Check sheet for the drawn part. Datum: minimum x, y, z corner. Units: mm. Round coordinates to 2 decimals unless told otherwise and drop trailing zeros. Order: outer loops, then holes, each group sorted by start corner. A loop starts at its lowest first (then second) coordinate and runs counter-clockwise, first axis right, second up. Notation, with made-up numbers: M 34.25,34 L 60.25,34 A20 cw 60.25,62 Z; hole C 41.25,78 d2. An arc over 180 degrees is marked long. Answer as a JSON object with one key per item and string values. Group by question number.
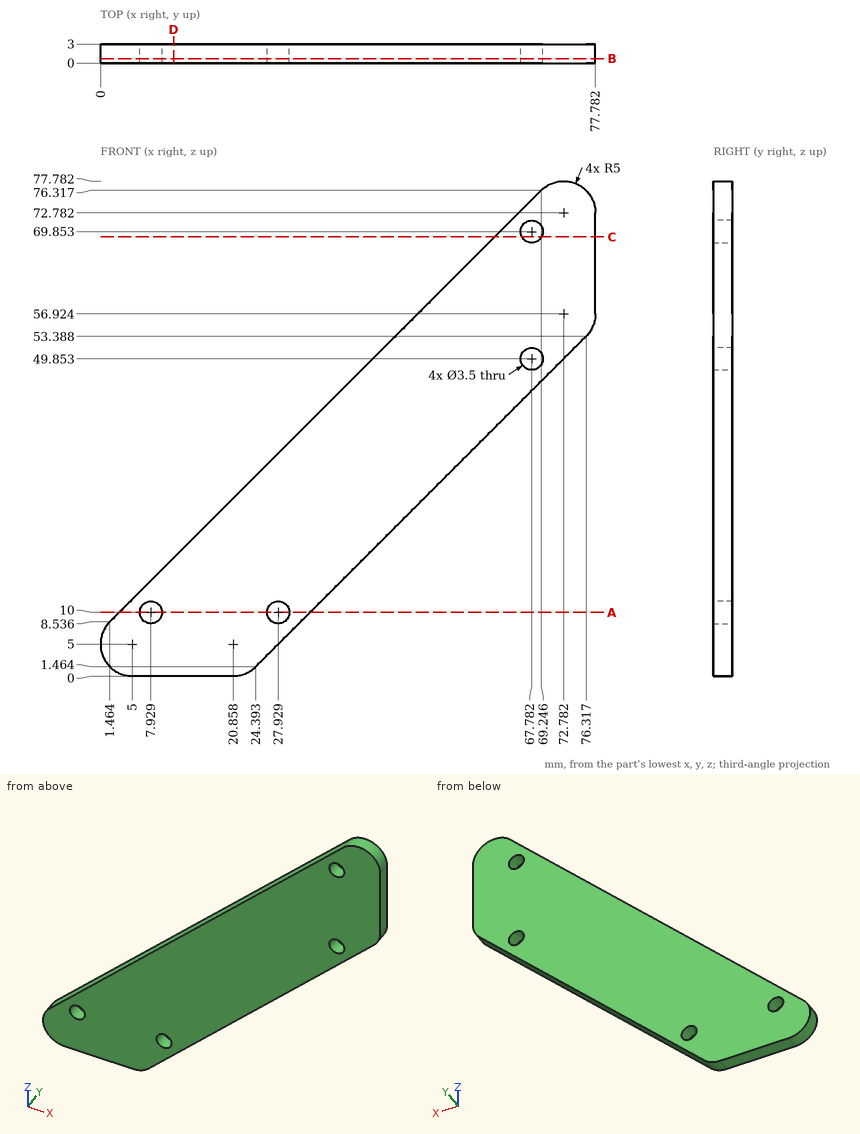
1) Thickness scan on line 1 along X through (y, z) = (1.9, 10); line 2 along Z through (x, y) = (8, 2.05); line 3 along Z through (x, y) = (27, 1.9) (1 decimal). Record the ranges inside material, lowest first. Write a range as [from, to].
2) Sectioned sample at A-A (z = 10). Record the boundary of the cut face in (x, y).
3) Sectioned sample at B-B (y = 0.7). Count the separate pieces of the cut face and the enclosed holes in it, then the cut area to 3 significant figures.
4) Sectioned sample at C-C (z = 69). Record the boundary of the cut face in (x, y), then the cut area to 3 significant figures.
5) Go/stop test with flat-tipped pins: P1, Ø3, axis at x = 7.93, z = 10, coming from the +Y side; P2, Ø12, axis at x = 41, z = 50, coming from the +Y side; P3, Ø1, axis at y = 0.5, z = 39, coming from the -X side. Record where each tip stops, or that it passes through.
6) Sectioned sample at D-D (x = 11.5). Record the boundary of the cut face in (y, z).
Final values:
{
 "1": {"line 1": "x = [2.93, 6.18], [9.68, 26.18], [29.68, 32.93]", "line 2": "z = [0, 8.25], [11.75, 15.07]", "line 3": "z = [4.1, 8.5], [11.5, 34.1]"},
 "2": {"outline": "M 2.93,0 L 6.18,0 L 6.18,3 L 2.93,3 Z; M 9.68,0 L 26.18,0 L 26.18,3 L 9.68,3 Z; M 29.68,0 L 32.93,0 L 32.93,3 L 29.68,3 Z"},
 "3": {"separate pieces": "1", "enclosed holes": "4", "area": "1,990 mm^2"},
 "4": {"outline": "M 61.93,0 L 66.25,0 L 66.25,3 L 61.93,3 Z; M 69.31,0 L 77.78,0 L 77.78,3 L 69.31,3 Z", "area": "38.4 mm^2"},
 "5": {"P1": "passes through", "P2": "stops at y = 3", "P3": "stops at x = 31.43"},
 "6": {"outline": "M 0,0 L 3,0 L 3,18.57 L 0,18.57 Z"}
}
